Verification items for the finished model (mm, model axes). A direction names the side the tool comes from. Give positions to 0.01 mm unless a question says otherwise; leave off trailing zeros. Loops run counter-clockwise (first coordinate to the right, second up) from the corner with the lowest first, then second, coordinate; pieces in that order, holes last. Notation, with made-up numbers: (-32, -15) -> (-25, -15) arc R26 ccw to (-25, 8) -> close; hole circle Ø2 at (23.25, 64). An arc over 180 degrees is marked (long way). Answer in a Markdown table with one row per item. Add a question column.
Q1. Section check A-A on y = 4. Enter the section's corners in (x, z) (3 decimals), and give its area (3 significant figures).
Q2. Material ranges on probe 1 along X at (y, z) = (1.5, 14) (3 decimals); probe 2 along X at (y, z) = (1, 10); probe 3 along Y at (x, z) = (9, 8.5), recorded low to high.
Q3. Release check for a two-part mould opening along X. For faces 1 (the face through (-14.605, 4, 19)), 2 (the face through (0, 11, 3.048)), 3 (the face through (-16.002, 6, 19)), 4 (the face through (-14.22, 8.53, 18.83)) record: pulls with the +X half, pulls with the -X half, needs draft (parallel to the pull), parting line crosses it, or undercut.
Q4. Gauge pin test, flat ends, axial feed: P1, Ø0.6, axis at x = 17, y = 1, coming from the +Z side; P2, Ø6, axis at y = 2.5, z = 8, coming from the +X side; P3, Ø3, axis at x = -2.5, z = 16.5, coming from the +Y side. Record the tip position at first contact, or that the pin passes through.
Q5. Set-up check for faces 5 (the face through (0, 11, 35.052)), 6 (the face through (14.605, 4, 19)): record each of +Z, -Z, +X, -X, +Y, -Y from which the full face is reachable in a straight line by a thin tool's end or side.
```python
from build123d import *

# Parameters (mm, degrees)
SKETCH1_RX              = 22.86
SKETCH1_RY              = 15.24
BOSS_EXTRUDE4_DEPTH     = 45.72
CUT_EXTRUDE2_START      = -10.16
SKETCH4_W               = 29.21
SKETCH4_H               = 17.78
CUT_EXTRUDE2_DEPTH      = 33.02
CUT_EXTRUDE4_DEPTH      = 33.02
CUT_EXTRUDE4_DEPTH_BACK = 33.02
SKETCH7_W               = 14.643913221
SKETCH7_H               = 35.56
SKETCH8_R               = 1.75
CUT_EXTRUDE5_DEPTH      = 1.27
SKETCH9_R               = 0.5
CUT_EXTRUDE7_DEPTH      = 2.794
FILLET1_R               = 1.27
FILLET2_R               = 1.27
SKETCH10_W              = 45.72
SKETCH10_H              = 17.78
CUT_EXTRUDE8_DEPTH      = 47.972834865
CUT_EXTRUDE10_START     = -15.24
CUT_EXTRUDE10_OUTLINE_W = 48
CUT_EXTRUDE10_OUTLINE_H = 38.1
CUT_EXTRUDE10_DEPTH     = 15.24
SKETCH15_W              = 29.21
SKETCH15_H              = 0.508
CUT_EXTRUDE13_DEPTH     = 42.866874941
SKETCH16_W              = 32.004
SKETCH16_H              = 0.3556
CUT_EXTRUDE14_DEPTH     = 39.891871036
BOSS_EXTRUDE5_START     = -10.16
SKETCH17_W              = 1.27
SKETCH17_H              = 1.27
BOSS_EXTRUDE5_DEPTH     = 12.7
FILLET3_R               = 0.762
FILLET4_R               = 0.762
FILLET5_R               = 0.762
FILLET6_R               = 1.27


# Read off the part's stored shape, not the designer's step: Cut-Extrude10
with BuildPart() as part:
    # Sketch1 → Boss-Extrude4 (new body)
    with BuildSketch(Plane.XY):
        with Locations(Location((0, 0), (0, 0, 180))):
            Ellipse(SKETCH1_RX, SKETCH1_RY)
    extrude(amount=BOSS_EXTRUDE4_DEPTH)

    # Sketch4 → Cut-Extrude2 (cut)
    with BuildSketch(Plane.XY.offset(45.72).offset(CUT_EXTRUDE2_START)):
        Rectangle(SKETCH4_W, SKETCH4_H)
    extrude(amount=-CUT_EXTRUDE2_DEPTH, mode=Mode.SUBTRACT)

    # Sketch7 → Cut-Extrude4 (cut, two sides: drawn at the far end of the back side and taken through both)
    with BuildSketch(Plane(origin=(0, 0, 0), x_dir=(0, 0, -1), z_dir=(1, 0, 0)).offset(-CUT_EXTRUDE4_DEPTH_BACK)):
        with Locations((-45.421956611, -1.677648267)):
            Rectangle(SKETCH7_W, SKETCH7_H)
    extrude(amount=CUT_EXTRUDE4_DEPTH + CUT_EXTRUDE4_DEPTH_BACK, mode=Mode.SUBTRACT)

    # Sketch8 → Cut-Extrude5 (cut)
    with BuildSketch(Plane.XY):
        Circle(SKETCH8_R)
        with Locations((4.064, 0)):
            Circle(SKETCH8_R)
        with Locations((-4.064, 0)):
            Circle(SKETCH8_R)
    extrude(amount=CUT_EXTRUDE5_DEPTH, mode=Mode.SUBTRACT)

    # Sketch9 → Cut-Extrude7 (cut)
    with BuildSketch(Plane(origin=(0, 0, 0), x_dir=(-1, 0, 0), z_dir=(0, 0, -1))):
        with Locations(Location((0, 0.8, 0), (0, 0, 180))):
            Circle(SKETCH9_R)
        with Locations(Location((0, -0.8, 0), (0, 0, 180))):
            Circle(SKETCH9_R)
        with Locations(Location((-4.064, 0.8, 0), (0, 0, 180))):
            Circle(SKETCH9_R)
        with Locations(Location((-4.064, -0.8, 0), (0, 0, 180))):
            Circle(SKETCH9_R)
        with Locations(Location((4.064, 0.8, 0), (0, 0, 180))):
            Circle(SKETCH9_R)
        with Locations(Location((4.064, -0.8, 0), (0, 0, 180))):
            Circle(SKETCH9_R)
    extrude(amount=-CUT_EXTRUDE7_DEPTH, mode=Mode.SUBTRACT)

    # Fillet1
    fillet1_edges = [part.edges().sort_by_distance(p)[0] for p in [
        (22.859987041, 0.016227247, 0),
    ]]
    fillet(fillet1_edges, radius=FILLET1_R)

    # Fillet2
    fillet2_edges = [part.edges().sort_by_distance(p)[0] for p in [
        (22.860000074, 1.7e-08, 38.1),
    ]]
    fillet(fillet2_edges, radius=FILLET2_R)

    # Sketch10 → Cut-Extrude8 (cut, through all)
    with BuildSketch(Plane(origin=(0, 0, 0), x_dir=(-1, 0, 0), z_dir=(0, 0, -1))):
        with Locations((0, -8.89)):
            Rectangle(SKETCH10_W, SKETCH10_H)
    extrude(amount=-CUT_EXTRUDE8_DEPTH, mode=Mode.SUBTRACT)

    # Cut-Extrude10 outline → Cut-Extrude10 (cut)
    with BuildSketch(Plane.XZ.offset(CUT_EXTRUDE10_START)):
        with Locations((0, 19.05)):
            Rectangle(CUT_EXTRUDE10_OUTLINE_W, CUT_EXTRUDE10_OUTLINE_H)
        Polygon((-16.002, 3.048), (-16.002, 35.052), (-14.605, 35.052), (-14.605, 35.56), (14.605, 35.56), (14.605, 35.052), (16.002, 35.052), (16.002, 3.048), (14.605, 3.048), (14.605, 2.54), (-14.605, 2.54), (-14.605, 3.048), align=None, mode=Mode.SUBTRACT)
    extrude(amount=CUT_EXTRUDE10_DEPTH, mode=Mode.SUBTRACT)

    # Sketch15 → Cut-Extrude13 (cut, through all)
    with BuildSketch(Plane(origin=(0, 0, 0), x_dir=(1, 0, 0), z_dir=(0, 1, 0))):
        with Locations((0, -2.794)):
            Rectangle(SKETCH15_W, SKETCH15_H)
        with Locations((0, -35.306)):
            Rectangle(SKETCH15_W, SKETCH15_H)
    extrude(amount=CUT_EXTRUDE13_DEPTH, mode=Mode.SUBTRACT)

    # Sketch16 → Cut-Extrude14 (cut, through all)
    with BuildSketch(Plane(origin=(0, 0, 3.048), x_dir=(-1, 0, 0), z_dir=(0, 0, -1))):
        with Locations((0, 0.1778)):
            Rectangle(SKETCH16_W, SKETCH16_H)
    extrude(amount=-CUT_EXTRUDE14_DEPTH, mode=Mode.SUBTRACT)

    # Sketch17 → Boss-Extrude5 (add)
    with BuildSketch(Plane(origin=(0, 0, 3.048), x_dir=(-1, 0, 0), z_dir=(0, 0, -1)).offset(BOSS_EXTRUDE5_START)):
        with Locations((-16.637, 0.9906)):
            Rectangle(SKETCH17_W, SKETCH17_H)
        with Locations((16.637, 0.9906)):
            Rectangle(SKETCH17_W, SKETCH17_H)
    extrude(amount=-BOSS_EXTRUDE5_DEPTH)

    # Fillet3
    fillet3_edges = [part.edges().sort_by_distance(p)[0] for p in [
        (16.002, 0.9906, 25.908),
        (16.002, 1.6256, 19.558),
        (16.002, 0.9906, 13.208),
    ]]
    fillet(fillet3_edges, radius=FILLET3_R)

    # Fillet4
    fillet4_edges = [part.edges().sort_by_distance(p)[0] for p in [
        (-16.002, 0.9906, 25.908),
        (-16.002, 1.6256, 19.558),
        (-16.002, 0.9906, 13.208),
    ]]
    fillet(fillet4_edges, radius=FILLET4_R)

    # Fillet5
    fillet5_edges = [part.edges().sort_by_distance(p)[0] for p in [
        (-14.605, 0.3556, 19.05),
        (14.605, 0.3556, 19.05),
    ]]
    fillet(fillet5_edges, radius=FILLET5_R)

    # Fillet6
    fillet6_edges = [part.edges().sort_by_distance(p)[0] for p in [
        (14.605, 8.89, 19.05),
        (-14.605, 8.89, 19.05),
    ]]
    fillet(fillet6_edges, radius=FILLET6_R)


solid = part.part
```
Taken from the geometry:
| question | item | result |
|---|---|---|
| 1 | outline | (-16.002, 3.048) -> (-14.605, 3.048) -> (-14.605, 35.052) -> (-16.002, 35.052) -> close; (14.605, 3.048) -> (16.002, 3.048) -> (16.002, 35.052) -> (14.605, 35.052) -> close |
| 1 | area | 89.4 mm² |
| 2 | probe 1 | x = -17.272 to -14.605, 14.605 to 17.272 |
| 2 | probe 2 | x = -16 to -14.61, 14.61 to 16 |
| 2 | probe 3 | y = 8.89 to 14.01 |
| 3 | face 1 | undercut |
| 3 | face 2 | needs draft |
| 3 | face 3 | pulls with the -X half |
| 3 | face 4 | undercut |
| 4 | P1 | stops at z = 25.91 |
| 4 | P2 | stops at x = 16 |
| 4 | P3 | stops at y = 15.23 |
| 5 | face 5 | +Z, +X, -X, +Y, -Y |
| 5 | face 6 | +Z, -Z, -Y |
